```python
from build123d import *

# Parameters (mm, degrees)
SKETCH1_W           = 4
SKETCH1_H           = 100
BOSS_EXTRUDE1_DEPTH = 80
SKETCH6_W           = 4
SKETCH6_H           = 12
BOSS_EXTRUDE2_DEPTH = 35
SKETCH14_R          = 12.5
SKETCH14_R_2        = 10.775
BOSS_EXTRUDE3_DEPTH = 12


with BuildPart() as part:
    # Sketch1 → Boss-Extrude1 (new body)
    with BuildSketch(Plane(origin=(10.75, 0, 0), x_dir=(0, 0, -1), z_dir=(1, 0, 0))):
        with Locations((0, 62)):
            Rectangle(SKETCH1_W, SKETCH1_H)
    extrude(amount=BOSS_EXTRUDE1_DEPTH)

    # Sketch6 → Boss-Extrude2 (add)
    with BuildSketch(Plane.ZY.offset(-10.75)):
        with Locations((0, 6)):
            Rectangle(SKETCH6_W, SKETCH6_H)
    extrude(amount=-BOSS_EXTRUDE2_DEPTH)

    # Sketch7 → Loft3 section 0
    with BuildSketch(Plane(origin=(45.75, 0, 0), x_dir=(0, 0, -1), z_dir=(1, 0, 0))):
        with BuildLine():
            Line((-2, 12), (2, 12))
            Line((2, 12), (2, 0))
            Line((2, 0), (-2, 0))
            Line((-2, 0), (-2, 12))
        make_face()
    # Sketch5 → Loft3 section 1
    with BuildSketch(Plane(origin=(90.75, 0, 0), x_dir=(0, 0, -1), z_dir=(1, 0, 0))):
        with BuildLine():
            Line((-2, 12), (2, 12))
            add(Edge.make_bspline(
                [(2, 12), (16.438366027, 4.561354626), (32, 0)],
                knots=[0, 0, 0, 1, 1, 1], degree=2))
            Line((32, 0), (-32, 0))
            add(Edge.make_bspline(
                [(-2, 12), (-16.438366027, 4.561354626), (-32, 0)],
                knots=[0, 0, 0, 1, 1, 1], degree=2))
        make_face()
    loft()


with BuildPart() as body_2:
    # Mirror3: mirrored copy
    add(part.part.mirror(Plane(origin=(0, 0, 0), x_dir=(0, 0, 1), z_dir=(1, 0, 0))))


with BuildPart() as part_1:
    add(part.part)

    add(body_2.part)  # Boss-Extrude3 merges body 2
    # Sketch14 → Boss-Extrude3 (add)
    with BuildSketch(Plane(origin=(0, 0, 0), x_dir=(1, 0, 0), z_dir=(0, 1, 0))):
        Circle(SKETCH14_R)
        Circle(SKETCH14_R_2, mode=Mode.SUBTRACT)
    extrude(amount=BOSS_EXTRUDE3_DEPTH)


solid = part_1.part
```
Can you work these out from the model? Positions are in its coordinate system, mm. A direction names the side the tool comes from. Coordinates: 2 decimals unless noted, no trailing zeros. Write each loop counter-clockwise with the first axis right and the second up, starting at its lowest first coordinate (ties: lowest second). Pieces come first, ordered by that corner, then holes. Notation, with made-up numbers: M 18,-39 L 42,-39 A18 cw 42,-10 Z; hole C 34,78.25 d2. An arc over 180 degrees is marked long. Write item = value, one per line. Start each with the question number.
Q1. On a 3-axis mill with a long thin cutter (end or side, diameter ignored), from which of +Z, -Z, +X, -X, +Y, -Y can I reach the whole of each face in a straight line? I mean faces 5 (the face through (0.227, 5.916, -10.773)), 6 (the face through (0.2, 5.9, -12.5)). Say none if no direction works.
Q2. If we section it at C-C, the plane z = 8.5: State how many separate pieces and enclosed holes the cut face has, then the cut area to 3 significant figures.
Q3. Thinking about a two-plate mould opening in X: for faces 1 (the face through (-90.75, 37, 0)), 2 (the face through (-0.227, 5.916, 10.773)), 3 (the face through (-10.75, 57, 0)), 4 (the face through (50, 112, 0)), which applies, released by +X, released by -X, zero draft, split by the parting line, or undercut?
Q4. If we section it at A-A, the plane y = 63: Write out the boundary of the cut face in (x, z), then the cut area to 3 significant figures.
Q5. I'm going to push flat-ended pins straight in: pin 1 (2 mm diameter, centred on x = -20.5, y = 69.5, fed in from +Z); pin 2 (8 mm diameter, centred on x = -13.5, y = 52, fed in from -Z); pin 3 (6 mm diameter, centred on x = 2, z = -9.5, fed in from +Y). Where does each tip first touch, or does it pass through?
Q6. If we section it at B-B, the plane x = 0: Write out the boundary of the cut face in (y, z) (3 decimals), then the cut area to 3 significant figures.
Q7. If I drill on L1, parallel to X at y = 96, z = 1; L2, parallel to Z at x = 12, y = 85; L3, parallel to X at y = 10.5, z = -8.5, over which ranges is the centre line in solid material (lowest first)? Write a range as [from, to].
Check sheet entries:
q1.face_5 = +Y, -Y
q1.face_6 = -Z, +Y, -Y
q2.separate_pieces = 4
q2.enclosed_holes = 0
q2.area = 517 mm²
q3.face_1 = released by -X
q3.face_2 = undercut
q3.face_3 = undercut
q3.face_4 = zero draft
q4.outline = M -90.75,-2 L -10.75,-2 L -10.75,2 L -90.75,2 Z; M 10.75,-2 L 90.75,-2 L 90.75,2 L 10.75,2 Z
q4.area = 640 mm²
q5.pin_1 = 2
q5.pin_2 = -2
q5.pin_3 = 12
q6.outline = M 0,-12.5 L 12,-12.5 L 12,-10.775 L 0,-10.775 Z; M 0,10.775 L 12,10.775 L 12,12.5 L 0,12.5 Z
q6.area = 41.4 mm²
q7.L1 = [-90.75, -10.75], [10.75, 90.75]
q7.L2 = [-2, 2]
q7.L3 = [-9.17, -6.62], [6.62, 9.17]
